The listing builds one solid part. Answer for the finished solid, in the listing's coordinates (mm). Face numbers are marked on the shaded views. A direction names the side the tool comes from. Coordinates: 2 decimals unless noted, no trailing zeros. Order: outer loops, then holes, each group sorted by start corner. A loop starts at its lowest first (then second) coordinate and runs counter-clockwise, first axis right, second up. Notation, with made-up numbers: M -18,23.5 L 13,23.5 A17 ccw 13,43.5 Z; hole C 53,-27 d8. An arc over 180 degrees is marked long. One line per item, written item: value. Start each with the question number.
Q1. The part is cut by section A-A on y = 0.85. Give the vertices of the cut face in (x, z), then the cut area to 3 significant figures.
Q2. Determine the mould class of the marked faces 1, 2 and 3 for opening direction X: pulls with the +X half, pulls with the -X half, needs draft (parallel to the pull), parting line crosses it, or undercut.
Q3. The part is cut by section B-B on y = 2.85. Give the vertices of the cut face in (x, z), then the cut area to 3 significant figures.
Q4. For the marked faces 4 and 5, determine the directions among +Z, -Z, +X, -X, +Y, -Y from which every point of the face is accessible in a straight line to the end or side of a thin tool.
Q5. Each of these flat-tipped pins is pushed along its axis until it touches: pin 1 Ø1.5 at (x, y) = (2.5, -1) entering from +Z; pin 2 Ø1 at (x, y) = (-2, -0.5) entering from +Z; pin 3 Ø2 at (x, y) = (-3, -0.5) entering from +Z. Where does it stop, or does it pass through?
Q6. Straight lines are drawn through the part: line 1 along X through (y, z) = (-0.55, 0); line 2 along Z through (x, y) = (2.5, 1.9); line 3 along Z through (x, y) = (-1.5, 1.2). For each, find the intervals that lie inside material, in ascending order. Write a range as [from, to].
```python
from build123d import *

# Parameters (mm, degrees)
BODYS_R             = 3
BODY_DEPTH          = 1.75
CHAMFERS_OUTSIDE_W  = 55.182
CHAMFERS_OUTSIDE_H  = 57.038
CHAMFERS_OUTSIDE_R  = 6
CHAMFER_2_DEPTH     = 10.810708435
CHAMFER_2_DRAFT     = -60
CM_COPY_1_SKETCH_W  = 55.182
CM_COPY_1_SKETCH_H  = 57.038
CM_COPY_1_SKETCH_R  = 6
CM_COPY_1_DEPTH     = 10.810708435
CM_COPY_1_DRAFT     = -60
FASTENINGBASES_R    = 6
FASTENINGBASES_R_2  = 3
FASTENINGBASE_DEPTH = 1.5


with BuildPart() as part:
    # BodyS → Body (new, symmetric)
    with BuildSketch(Plane(origin=(0, 0, 0), x_dir=(1, 0, 0), z_dir=(0, 1, 0))):
        Polygon((-6, 3.464101615), (-6, -3.464101615), (0, -6.92820323), (6, -3.464101615), (6, 3.464101615), (0, 6.92820323), align=None)
        with Locations(Location((0, 0, 0), (0, 0, 270))):
            Circle(BODYS_R, mode=Mode.SUBTRACT)
    extrude(amount=BODY_DEPTH, both=True)


with BuildPart() as chamfer_2_tool:
    # ChamferS outside → Chamfer 2 (with draft: the straight prism first)
    with BuildSketch(Plane(origin=(0, 1.75, 0), x_dir=(1, 0, 0), z_dir=(0, 1, 0))):
        Rectangle(CHAMFERS_OUTSIDE_W, CHAMFERS_OUTSIDE_H)
        Circle(CHAMFERS_OUTSIDE_R, mode=Mode.SUBTRACT)
    extrude(amount=-CHAMFER_2_DEPTH)
    # Chamfer 2: the draft: its side faces are tilted about the plane it starts from
    chamfer_2_sides = [chamfer_2_tool.faces().sort_by_distance(p)[0] for p in [
        (0, -3.655354218, 28.519),
        (27.591, -3.655354218, 0),
        (0, -3.655354218, -28.519),
        (-27.591, -3.655354218, 0),
        (-6, -3.655354218, 0),
    ]]
    draft(chamfer_2_sides, Plane(origin=(0, 1.75, 0), x_dir=(1, 0, 0), z_dir=(0, 1, 0)), CHAMFER_2_DRAFT)


with BuildPart() as part_1:
    add(part.part)

    # Chamfer 2: cut by chamfer_2_tool
    add(chamfer_2_tool.part, mode=Mode.SUBTRACT)


with BuildPart() as cm_copy_1_tool:
    # CM copy 1 sketch → CM copy 1 (with draft: the straight prism first)
    with BuildSketch(Plane.XZ.offset(1.75)):
        Rectangle(CM_COPY_1_SKETCH_W, CM_COPY_1_SKETCH_H)
        Circle(CM_COPY_1_SKETCH_R, mode=Mode.SUBTRACT)
    extrude(amount=-CM_COPY_1_DEPTH)
    # CM copy 1: the draft: its side faces are tilted about the plane it starts from
    cm_copy_1_sides = [cm_copy_1_tool.faces().sort_by_distance(p)[0] for p in [
        (0, 3.655354218, 28.519),
        (27.591, 3.655354218, 0),
        (0, 3.655354218, -28.519),
        (-27.591, 3.655354218, 0),
        (-6, 3.655354218, 0),
    ]]
    draft(cm_copy_1_sides, Plane.XZ.offset(1.75), CM_COPY_1_DRAFT)


with BuildPart() as part_2:
    add(part_1.part)

    # CM copy 1: cut by cm_copy_1_tool
    add(cm_copy_1_tool.part, mode=Mode.SUBTRACT)

    # FasteningBaseS → FasteningBase (add)
    with BuildSketch(Plane(origin=(0, 1.75, 0), x_dir=(1, 0, 0), z_dir=(0, 1, 0))):
        with Locations(Location((0, 0, 0), (0, 0, 60))):
            Circle(FASTENINGBASES_R)
        with Locations(Location((0, 0, 0), (0, 0, 270))):
            Circle(FASTENINGBASES_R_2, mode=Mode.SUBTRACT)
    extrude(amount=FASTENINGBASE_DEPTH)


solid = part_2.part
```
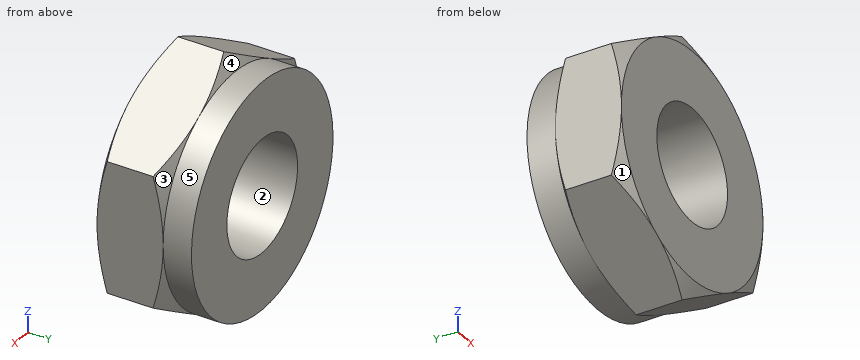
Output:
1. outline: M -6,-3.46 L 0,-6.93 L 6,-3.46 L 6,3.46 L 0,6.93 L -6,3.46 Z; hole C 0,0 d6
1. area: 96.4 mm^2
2. face 1: pulls with the -X half
2. face 2: undercut
2. face 3: pulls with the +X half
3. outline: C 0,0 d12; hole C 0,0 d6
3. area: 84.8 mm^2
4. face 4: +Z, +Y
4. face 5: +Y
5. pin 1: stops at z = 5.92
5. pin 2: stops at z = 6.06
5. pin 3: stops at z = 5.77
6. line 1: x = [-6, -3], [3, 6]
6. line 2: z = [-5.45, -1.66], [1.66, 5.45]
6. line 3: z = [-6.06, -2.6], [2.6, 6.06]
